Design review of the part shown in the three views and the two pictorial views. Dimensions are in mm from the part's minimum x, y and z. A direction names the side the tool comes from. Give positions to 0.01 mm unless a question says otherwise; leave off trailing zeros. Loops run counter-clockwise (first coordinate to the right, second up) from the corner with the lowest first, then second, coordinate; pieces in that order, holes last.
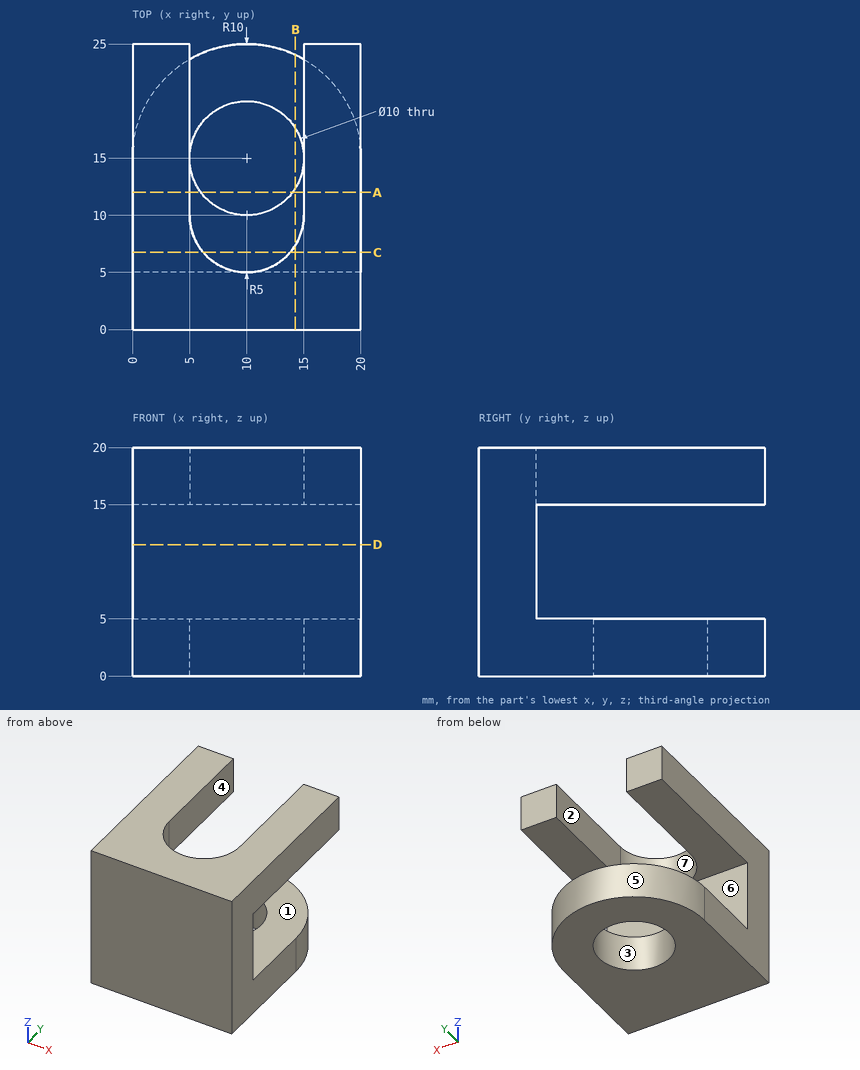
Q1. For pin 1 Ø1 at (x, y) = (2.5, 15.5) entering from -Z; pin 2 Ø3 at (x, z) = (8.5, 7.5) entering from +Y, all flat-tipped, find the tip position at first contact; note any pin that passes through.
Answers:
pin 1: stops at z = 0
pin 2: stops at y = 5
Q2. Consider section A-A on y = 12. Give the boundary of the cut face in (x, z), plus the area to 3 significant figures.
Answers:
outline: (0, 0) - (6, 0) - (6, 5) - (0, 5) - close; (0, 15) - (5, 15) - (5, 20) - (0, 20) - close; (14, 0) - (20, 0) - (20, 5) - (14, 5) - close; (15, 15) - (20, 15) - (20, 20) - (15, 20) - close
area: 110 mm2
Q3. Machinability: for the marked faces 1, 2 and 3, which of the approach directions +Z, -Z, +X, -X, +Y, -Y give a long, thin tool a straight path to every point of the face, cutting with its end or side? Answer none if there is none.
Answers:
face 1: +X, -X, +Y
face 2: +Z, +Y
face 3: +Z, -Z
Q4. For probe 1 along X at (y, z) = (11.5, 15.75); probe 2 along Y at (x, z) = (10, 1.9), list the stretches that pass through material, from the lowest coordinate up.
Answers:
probe 1: x = 0 to 5, 15 to 20
probe 2: y = 0 to 10, 20 to 25
Q5. Consider section C-C on y = 6.75. Give the boundary of the cut face in (x, z).
Answers:
outline: (0, 0) - (20, 0) - (20, 5) - (0, 5) - close; (0, 15) - (6.2, 15) - (6.2, 20) - (0, 20) - close; (13.8, 15) - (20, 15) - (20, 20) - (13.8, 20) - close
Q6. Consider section B-B on x = 14.25. Give the boundary of the cut face in (y, z).
Answers:
outline: (0, 0) - (12.37, 0) - (12.37, 5) - (5, 5) - (5, 15) - (7.37, 15) - (7.37, 20) - (0, 20) - close; (17.63, 0) - (24.05, 0) - (24.05, 5) - (17.63, 5) - close
Q7. Consider section D-D on z = 11.5. Give the boundary of the cut face in (x, y).
Answers:
outline: (0, 0) - (20, 0) - (20, 5) - (0, 5) - close
Q8. Mouldability with a two-part tool opening along X and no side actions: class the marked faces 4, 5, 6 and 7 as +X half, -X half, draft (parallel to the pull), parting line (faces both ways), or undercut.
Answers:
face 4: undercut
face 5: parting line
face 6: draft
face 7: undercut
